Verification items for the finished model (mm, model axes). A direction names the side the tool comes from. Coordinates: 2 decimals unless noted, no trailing zeros. Loops run counter-clockwise (first coordinate to the right, second up) from the corner with the lowest first, then second, coordinate; pieces in that order, holes last. Notation, with made-up numbers: M -34,3 L -27,3 A14 cw -27,22 Z; hole C -19.5,57.25 d5. An arc over 180 degrees is marked long. Write item = value, one per line. Start each with the question number.
```python
from build123d import *

# Parameters (mm, degrees)
F1_DEPTH = 25.4
F3_D     = 12.7


with BuildPart() as f1:
    # F0 (on Front) → F1 (new body)
    with BuildSketch(Plane.XZ):
        Polygon((0, -508), (0, 0), (0, 508), (-76.2, 508), (-76.2, 254), (-254, 76.2), (-508, 76.2), (-508, -76.2), (-254, -76.2), (-76.2, -254), (-76.2, -508), align=None)
        Polygon((0, 508), (0, 0), (508, 0), (508, 76.2), (254, 76.2), (76.2, 254), (76.2, 508), align=None)
        Polygon((508, 0), (0, 0), (0, -508), (76.2, -508), (76.2, -254), (254, -76.2), (508, -76.2), align=None)
    extrude(amount=F1_DEPTH)

    # F3 (through all)
    with Locations(Plane.XZ.offset(25.4)):
        with Locations((0, 444.5), (0, 254), (254, 0), (444.5, 0), (0, -254), (0, -444.5), (-254, 0), (-444.5, 0)):
            Hole(F3_D / 2)


solid = f1.part
```
Q1. Sectioned sample at B-B on x = -211. Record the cut outline in (y, z), plus the area to 3 significant figures.
Q2. Scan lines: L1, parallel to Z at x = -254, y = -15.5; L2, parallel to Z at x = 0, y = -7.5. Record each from-to range of solid material in increasing order. Write a range as [from, to].
Q3. Gauge pin test, flat ends, axial feed: pin 1 (7.5 mm diameter, centred on x = 0, z = -254, fed in from +Y); pin 2 (7.5 mm diameter, centred on y = -14, z = -357.5, fed in from -X); pin 3 (8 mm diameter, centred on x = -101, y = -3, fed in from -Z); pin 4 (3 mm diameter, centred on y = -11, z = -101, fed in from +X). Record the tip position at first contact, or that the pin passes through.
Q4. Set-up check for faces 1 (the face through (379, -13, -76.2)), 2 (the face through (-379, -13, 76.2)), 3 (the face through (383, -13, 76.2)): record each of +Z, -Z, +X, -X, +Y, -Y from which the full face is reachable in a straight line by a thin tool's end or side.
Q5. Sectioned sample at C-C on z = 281.5. Record the cut outline in (x, y), plus the area to 3 significant figures.
Q6. Sectioned sample at A-A on y = -11.75. Count the separate pieces of the cut face and the enclosed holes in it, plus the area to 3 significant figures.
Solutions:
q1.outline = M -25.4,-119.2 L 0,-119.2 L 0,119.2 L -25.4,119.2 Z
q1.area = 6,060 mm²
q2.L1 = [-76.2, -6.35], [6.35, 76.2]
q2.L2 = [-508, -450.85], [-438.15, -260.35], [-247.65, 247.65], [260.35, 438.15], [450.85, 508]
q3.pin_1 = through
q3.pin_2 = -76.2
q3.pin_3 = -233.2
q3.pin_4 = 230.7
q4.face_1 = -Z, +X, +Y, -Y
q4.face_2 = +Z, -X, +Y, -Y
q4.face_3 = +Z, +X, +Y, -Y
q5.outline = M -76.2,-25.4 L 76.2,-25.4 L 76.2,0 L -76.2,0 Z
q5.area = 3,870 mm²
q6.separate_pieces = 1
q6.enclosed_holes = 8
q6.area = 349,000 mm²
